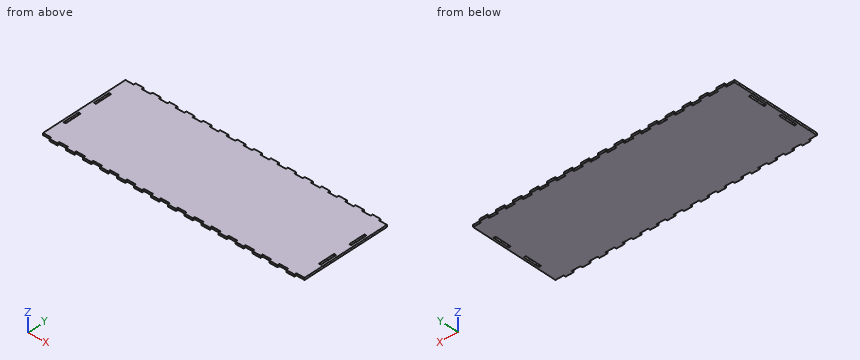
```python
from build123d import *

# Parameters (mm, degrees)
SKETCH1_W           = 3.175
SKETCH1_H           = 25.4
BOSS_EXTRUDE1_DEPTH = 3.175


with BuildPart() as part:
    # Sketch1 → Boss-Extrude1 (new body)
    with BuildSketch(Plane.XY):
        Polygon((406.4, 0), (406.4, 138.0236), (393.7, 138.0236), (393.7, 141.1986), (381, 141.1986), (381, 138.0236), (367.392857143, 138.0236), (367.392857143, 141.1986), (354.692857143, 141.1986), (354.692857143, 138.0236), (341.085714286, 138.0236), (341.085714286, 141.1986), (328.385714286, 141.1986), (328.385714286, 138.0236), (314.778571429, 138.0236), (314.778571429, 141.1986), (302.078571429, 141.1986), (302.078571429, 138.0236), (288.471428571, 138.0236), (288.471428571, 141.1986), (275.771428571, 141.1986), (275.771428571, 138.0236), (262.164285714, 138.0236), (262.164285714, 141.1986), (249.464285714, 141.1986), (249.464285714, 138.0236), (235.857142857, 138.0236), (235.857142857, 141.1986), (223.157142857, 141.1986), (223.157142857, 138.0236), (209.55, 138.0236), (209.55, 141.1986), (196.85, 141.1986), (196.85, 138.0236), (183.242857143, 138.0236), (183.242857143, 141.1986), (170.542857143, 141.1986), (170.542857143, 138.0236), (156.935714286, 138.0236), (156.935714286, 141.1986), (144.235714286, 141.1986), (144.235714286, 138.0236), (130.628571429, 138.0236), (130.628571429, 141.1986), (117.928571429, 141.1986), (117.928571429, 138.0236), (104.321428571, 138.0236), (104.321428571, 141.1986), (91.621428571, 141.1986), (91.621428571, 138.0236), (78.014285714, 138.0236), (78.014285714, 141.1986), (65.314285714, 141.1986), (65.314285714, 138.0236), (51.707142857, 138.0236), (51.707142857, 141.1986), (39.007142857, 141.1986), (39.007142857, 138.0236), (25.4, 138.0236), (25.4, 141.1986), (12.7, 141.1986), (12.7, 138.0236), (0, 138.0236), (0, 0), (12.7, 0), (12.7, -3.175), (25.4, -3.175), (25.4, 0), (39.007142857, 0), (39.007142857, -3.175), (51.707142857, -3.175), (51.707142857, 0), (65.314285714, 0), (65.314285714, -3.175), (78.014285714, -3.175), (78.014285714, 0), (91.621428571, 0), (91.621428571, -3.175), (104.321428571, -3.175), (104.321428571, 0), (117.928571429, 0), (117.928571429, -3.175), (130.628571429, -3.175), (130.628571429, 0), (144.235714286, 0), (144.235714286, -3.175), (156.935714286, -3.175), (156.935714286, 0), (170.542857143, 0), (170.542857143, -3.175), (183.242857143, -3.175), (183.242857143, 0), (196.85, 0), (196.85, -3.175), (209.55, -3.175), (209.55, 0), (223.157142857, 0), (223.157142857, -3.175), (235.857142857, -3.175), (235.857142857, 0), (249.464285714, 0), (249.464285714, -3.175), (262.164285714, -3.175), (262.164285714, 0), (275.771428571, 0), (275.771428571, -3.175), (288.471428571, -3.175), (288.471428571, 0), (302.078571429, 0), (302.078571429, -3.175), (314.778571429, -3.175), (314.778571429, 0), (328.385714286, 0), (328.385714286, -3.175), (341.085714286, -3.175), (341.085714286, 0), (354.692857143, 0), (354.692857143, -3.175), (367.392857143, -3.175), (367.392857143, 0), (381, 0), (381, -3.175), (393.7, -3.175), (393.7, 0), align=None)
        with Locations((4.7625, 94.4118)):
            Rectangle(SKETCH1_W, SKETCH1_H, mode=Mode.SUBTRACT)
        with Locations((4.7625, 43.6118)):
            Rectangle(SKETCH1_W, SKETCH1_H, mode=Mode.SUBTRACT)
        with Locations((401.6375, 43.6118)):
            Rectangle(SKETCH1_W, SKETCH1_H, mode=Mode.SUBTRACT)
        with Locations((401.6375, 94.4118)):
            Rectangle(SKETCH1_W, SKETCH1_H, mode=Mode.SUBTRACT)
    extrude(amount=BOSS_EXTRUDE1_DEPTH)


solid = part.part
```
Could you check a few things on this model? Use its own coordinates, in mm. Coordinates: 2 decimals unless noted, no trailing zeros. Write each loop counter-clockwise with the first axis right and the second up, starting at its lowest first coordinate (ties: lowest second). Pieces come first, ordered by that corner, then holes. Notation, with made-up numbers: (-14.5, -28) -> (31.5, -28) arc R23 ccw to (31.5, -19) -> close; hole circle Ø7 at (-8, 37.5). An arc over 180 degrees is marked (long way). Write item = value, one per line. Start each with the question number.
(1) I want a section at B-B (z = 2.25). Give the number of separate pieces and of enclosed holes in the cut face, plus the area to 3 significant figures.
(2) I need wall thicknesses on line 1 (X direction, y = 31.5, z = 0.2) (3 decimals); line 2 (Y direction, x = 219, z = 0.8). Which ranges of each line are inside material? Lowest first, please. Write a range as [from, to].
(3) I want a section at C-C (x = 292.5). Please give me the cut outline in (y, z) (3 decimals), plus the area to 3 significant figures.
(4) I want a section at A-A (y = 90). Please give me the cut outline in (x, z) (3 decimals).
(5) Will these pins go through, and if not, where does the flat tip stop? pin 1 (1.6 mm diameter, centred on y = -2, z = 1.5, fed in from +X); pin 2 (1 mm diameter, centred on x = 5, z = 1.5, fed in from -Y); pin 3 (1 mm diameter, centred on y = 140, z = 1.5, fed in from -X).
Result set:
q1.separate_pieces = 1
q1.enclosed_holes = 4
q1.area = 57,000 mm2
q2.line_1 = [0, 3.175], [6.35, 400.05], [403.225, 406.4]
q2.line_2 = [0, 138.02]
q3.outline = (0, 0) -> (138.024, 0) -> (138.024, 3.175) -> (0, 3.175) -> close
q3.area = 438 mm2
q4.outline = (0, 0) -> (3.175, 0) -> (3.175, 3.175) -> (0, 3.175) -> close; (6.35, 0) -> (400.05, 0) -> (400.05, 3.175) -> (6.35, 3.175) -> close; (403.225, 0) -> (406.4, 0) -> (406.4, 3.175) -> (403.225, 3.175) -> close
q5.pin_1 = 393.7
q5.pin_2 = 0
q5.pin_3 = 12.7
